Model file for the job. Use its own axes, mm. Give positions to 0.01 mm unless a question says otherwise; leave off trailing zeros. Write each loop counter-clockwise with the first axis right and the second up, starting at its lowest first coordinate (ties: lowest second). Pieces come first, ordered by that corner, then holes. Notation, with made-up numbers: (70.25, 46) - (75.25, 46) arc R28 ccw to (75.25, 79) - close; hole circle Ø10 at (72.5, 31.5). An arc over 180 degrees is marked (long way). Use CSV: the item, a comma, the result in double quotes.
Autodesk Inventor part; units mm, degrees
ref_plane "YZ Plane" through (0, 0, 0) normal (1, 0, 0) x (0, 1, 0)
ref_plane "XZ Plane" through (0, 0, 0) normal (0, 1, 0) x (-1, 0, 0)
ref_plane "XY Plane" through (0, 0, 0) normal (0, 0, 1) x (1, 0, 0)
sketch "Sketch1" plane through (0, 0, 0) normal (0, 0, 1) x (1, 0, 0)
  line L0 (0, 0) -> (380, 0)
  line L1 (380, 0) -> (380, 380)
  line L2 (380, 380) -> (0, 380)
  line L3 (0, 380) -> (0, 0)
  dimension "d0" = 380
  dimension "d1" = 380
extrude "Extrusion1" add sketch "Sketch1" along normal blind 380
sketch "Sketch2" plane through (0, 0, 380) normal (0, 0, 1) x (1, 0, 0)
  line L0 (30, 350) -> (350, 350)
  line L1 (350, 350) -> (350, 30)
  line L2 (350, 30) -> (30, 30)
  line L3 (30, 30) -> (30, 350)
  line L4 (380, 380) -> (0, 380)
  line L5 (0, 380) -> (0, 0)
  line L6 (0, 0) -> (380, 0)
  line L7 (380, 0) -> (380, 380)
  dimension "d4" = 30
  dimension "d5" = 30
  dimension "d6" = 30
  dimension "d7" = 30
extrude "Extrusion2" cut sketch "Sketch2" against normal blind 600 contours L0 L1 L2 L3
sketch "Sketch3" plane through (380, 0, 0) normal (1, 0, 0) x (0, 0, -1)
  line L0 (-350, 350) -> (-30, 350)
  line L1 (-30, 350) -> (-30, 30)
  line L2 (-30, 30) -> (-350, 30)
  line L3 (-350, 30) -> (-350, 350)
  line L4 (0, 380) -> (-380, 380)
  line L5 (-380, 0) -> (-380, 380)
  line L6 (0, 0) -> (0, 380)
  line L7 (0, 0) -> (-380, 0)
  dimension "d10" = 30
  dimension "d11" = 30
  dimension "d12" = 30
  dimension "d13" = 30
extrude "Extrusion3" cut sketch "Sketch3" against normal blind 600 contours L0 L1 L2 L3
sketch "Sketch4" plane through (0, 380, 0) normal (0, 1, 0) x (1, 0, 0)
  line L0 (30, -30) -> (30, 0)
  line L1 (350, -380) -> (350, -350)
  line L2 (30, -30) -> (350, -30)
  line L3 (350, -30) -> (350, -350)
  line L4 (350, -350) -> (30, -350)
  line L5 (30, -350) -> (30, -30)
  point P0 (0, 0)
extrude "Extrusion4" cut sketch "Sketch4" against normal blind 600
sketch "Sketch5" plane through (30, 0, 30) normal (1, 0, 0) x (0, 0, -1)
  line L0 (-350, 30) -> (-320, 30)
  line L1 (0, 30) -> (0, 0)
  line L2 (-320, 30) -> (0, 30)
  line L3 (0, 30) -> (0, 0)
  line L4 (0, 0) -> (-320, 0)
  line L5 (-320, 0) -> (-320, 30)
  point P0 (30, 0)
extrude "Extrusion5" add sketch "Sketch5" along normal blind 15
sketch "Sketch6" plane through (350, 0, 30) normal (0, 0, 1) x (1, 0, 0)
  line L0 (-320, 30) -> (-350, 30)
  line L1 (0, 30) -> (0, 0)
  line L2 (-320, 30) -> (0, 30)
  line L3 (0, 30) -> (0, 0)
  line L4 (0, 0) -> (-320, 0)
  line L5 (-320, 0) -> (-320, 30)
  point P0 (-350, 0)
extrude "Extrusion6" add sketch "Sketch6" along normal blind 15
sketch "Sketch7" plane through (350, 0, 350) normal (-1, 0, 0) x (0, 0, 1)
  line L0 (0, 30) -> (-320, 30)
  line L1 (0, 0) -> (-305, 0)
  line L2 (-320, 30) -> (0, 30)
  line L3 (0, 30) -> (0, 0)
  line L4 (0, 0) -> (-320, 0)
  line L5 (-320, 0) -> (-320, 30)
  point P0 (-350, 0)
extrude "Extrusion7" add sketch "Sketch7" along normal blind 15
sketch "Sketch8" plane through (45, 0, 350) normal (0, 0, -1) x (-1, 0, 0)
  line L0 (45, 0) -> (-335, 0)
  line L1 (-305, 30) -> (15, 30)
  line L2 (15, 30) -> (15, 0)
  line L3 (15, 0) -> (-305, 0)
  line L4 (-305, 0) -> (-305, 30)
  dimension "d24" = 320
extrude "Extrusion8" add sketch "Sketch8" along normal blind 15
sketch "Sketch9" plane through (0, 380, 0) normal (0, 1, 0) x (1, 0, 0)
  line L0 (0, -380) -> (380, -380)
  line L1 (0, 0) -> (20, 0)
  line L2 (10, -380) -> (0, -380)
  line L3 (0, -380) -> (0, 0)
  line L4 (20, 0) -> (380, 0)
  line L5 (380, 0) -> (380, -10)
  line L6 (380, -10) -> (10, -10)
  line L7 (10, -10) -> (10, -380)
  line L8 (0, -30) -> (0, -350)
  dimension "d27" = 10
  dimension "d28" = 10
extrude "Extrusion9" cut sketch "Sketch9" against normal blind 900
sketch "Sketch10" plane through (10, 380, 10) normal (0, 1, 0) x (1, 0, 0)
  line L0 (370, 0) -> (360, 0)
  line L1 (360, 0) -> (360, -370)
  line L2 (360, -370) -> (370, -370)
  line L3 (370, -370) -> (370, 0)
  line L4 (0, -370) -> (360, -370)
  line L5 (360, -370) -> (360, -360)
  line L6 (360, -360) -> (0, -360)
  line L7 (0, -360) -> (0, -370)
  point P0 (-10, 10)
  dimension "d31" = 10
  dimension "d32" = 10
extrude "Extrusion10" cut sketch "Sketch10" against normal blind 900
sketch "Sketch11" plane through (370, 380, 370) normal (1, 0, 0) x (0, 0, -1)
  line L0 (0, 0) -> (360, 0)
  line L1 (0, 0) -> (360, 0)
  line L2 (360, 0) -> (360, -10)
  line L3 (360, -10) -> (0, -10)
  line L4 (0, -10) -> (0, 0)
  line L5 (360, 0) -> (360, -380)
  line L6 (0, -380) -> (360, -380)
  line L7 (360, -380) -> (360, -370)
  line L8 (360, -370) -> (0, -370)
  line L9 (0, -370) -> (0, -380)
  point P0 (370, -380)
  dimension "d35" = 10
  dimension "d36" = 10
extrude "Extrusion11" cut sketch "Sketch11" against normal blind 900
sketch "Sketch13" plane through (10, 10, 370) normal (0, 0, 1) x (1, 0, 0)
  line L0 (0, 0) -> (360, 0)
  line L1 (360, 0) -> (260, 0)
  line L2 (260, 0) -> (260, 500)
  line L3 (260, 500) -> (360, 500)
  line L4 (360, 500) -> (360, 0)
  point P0 (-10, -10)
  point P1 (260, 0)
  dimension "d41" = 100
  dimension "d42" = 500
extrude "Extrusion13" add sketch "Sketch13" along normal blind 100
sketch "Sketch14" plane through (270, 510, 370) normal (0, 1, 0) x (1, 0, 0)
  line L0 (10, -10) -> (90, -10)
  line L1 (90, -10) -> (90, -90)
  line L2 (90, -90) -> (10, -90)
  line L3 (10, -90) -> (10, -10)
  line L4 (100, 0) -> (0, 0)
  line L5 (0, 0) -> (0, -100)
  line L6 (100, -100) -> (0, -100)
  line L7 (100, 0) -> (100, -100)
  point P0 (-270, 370)
  dimension "d45" = 10
  dimension "d46" = 10
  dimension "d47" = 10
  dimension "d48" = 10
extrude "Extrusion14" cut sketch "Sketch14" against normal blind 900 contours L0 L1 L2 L3
sketch "Sketch15" plane through (10, 10, 470) normal (0, 0, 1) x (1, 0, 0)
  line L0 (270, 500) -> (270, 0)
  line L1 (360, 20) -> (340, 20)
  line L2 (270, 490) -> (350, 490)
  line L3 (350, 490) -> (350, 20)
  line L4 (350, 20) -> (270, 20)
  line L5 (270, 20) -> (270, 490)
  line L6 (360, 500) -> (260, 500)
  point P0 (-10, -10)
  point P1 (270, 20)
  dimension "d51" = 10
extrude "Extrusion15" cut sketch "Sketch15" against normal blind 100
sketch "Sketch16" plane through (370, 10, 10) normal (1, 0, 0) x (0, 0, -1)
  line L0 (-450, 490) -> (-370, 490)
  line L1 (-370, 490) -> (-370, 20)
  line L2 (-370, 20) -> (-450, 20)
  line L3 (-450, 20) -> (-450, 490)
  line L4 (-360, 500) -> (-460, 500)
  line L5 (-460, 0) -> (-460, 500)
  line L6 (-360, 360) -> (-360, 500)
  line L7 (0, 0) -> (-460, 0)
  point P0 (10, -10)
  dimension "d54" = 10
  dimension "d55" = 10
  dimension "d56" = 10
  dimension "d57" = 20
extrude "Extrusion16" cut sketch "Sketch16" against normal blind 100
sketch "Sketch17" plane through (10, 10, 10) normal (0, -1, 0) x (1, 0, 0)
  line L0 (270, 450) -> (350, 450)
  line L1 (270, 370) -> (350, 370)
  line L2 (270, 450) -> (350, 450)
  line L3 (350, 450) -> (350, 370)
  line L4 (350, 370) -> (270, 370)
  line L5 (270, 370) -> (270, 450)
  point P0 (-10, -10)
  point P1 (350, 450)
extrude "Extrusion17" add sketch "Sketch17" against normal blind 20
sketch "Sketch19" plane through (370, 10, 10) normal (1, 0, 0) x (0, 0, -1)
  line L0 (-360, 500) -> (-460, 500)
  line L1 (-360, 490) -> (-360, 360)
  line L2 (-460, 500) -> (-360, 500)
  line L3 (-360, 500) -> (-360, 420)
  line L4 (-360, 420) -> (-460, 420)
  line L5 (-460, 420) -> (-460, 500)
  point P0 (10, -10)
  dimension "d65" = 80
extrude "Extrusion19" cut sketch "Sketch19" against normal blind 8900
sketch "Sketch20" plane through (370, 10, 10) normal (1, 0, 0) x (0, 0, -1)
  line L0 (-460, 420) -> (-450, 420)
  line L1 (-360, 360) -> (-360, 20)
  line L2 (-460, 420) -> (-360, 420)
  line L3 (-360, 420) -> (-360, 360)
  line L4 (-360, 360) -> (-460, 360)
  line L5 (-460, 360) -> (-460, 420)
  point P0 (10, -10)
extrude "Extrusion20" cut sketch "Sketch20" against normal blind 8900
sketch "Sketch21" plane through (270, 370, 380) normal (0, 0, 1) x (1, 0, 0)
  line L0 (10, -20) -> (10, 0)
  line L1 (0, 0) -> (10, 0)
  line L2 (10, 0) -> (10, -20)
  line L3 (10, -20) -> (0, -20)
  line L4 (0, -20) -> (0, 0)
  point P0 (-270, -370)
extrude "Extrusion21" add sketch "Sketch21" along normal up to surface (80 mm away)
sketch "Sketch22" plane through (280, 30, 470) normal (1, 0, 0) x (0, 0, -1)
  line L0 (0, 340) -> (10, 340)
  line L1 (10, 340) -> (10, 320)
  line L2 (10, 320) -> (0, 320)
  line L3 (0, 320) -> (0, 340)
  point P0 (470, -30)
  dimension "d72" = 20
extrude "Extrusion22" add sketch "Sketch22" along normal up to surface (80 mm away)
sketch "Sketch23" plane through (370, 10, 10) normal (1, 0, 0) x (0, 0, -1)
  line L0 (-370, 20) -> (-370, 360)
  line L1 (-450, 360) -> (-370, 360)
  line L2 (-370, 360) -> (-370, 340)
  line L3 (-370, 340) -> (-450, 340)
  line L4 (-450, 340) -> (-450, 360)
  point P0 (10, -10)
  dimension "d75" = 20
extrude "Extrusion23" add sketch "Sketch23" against normal blind 10
sketch "Sketch26" plane through (10, 10, 10) normal (0, -1, 0) x (1, 0, 0)
  line L0 (260, 460) -> (360, 460)
  line L1 (360, 0) -> (360, 460)
  line L2 (260, 460) -> (360, 460)
  line L3 (360, 460) -> (360, 360)
  line L4 (360, 360) -> (260, 360)
  line L5 (260, 360) -> (260, 460)
  point P0 (-10, -10)
  dimension "d86" = 100
extrude "Extrusion26" add sketch "Sketch26" along normal blind 120
sketch "Sketch30" plane through (10, 10, 470) normal (0, 0, 1) x (1, 0, 0)
  line L0 (360, 360) -> (260, 360)
  line L1 (260, 340) -> (260, 20)
  line L2 (360, 360) -> (260, 360)
  line L3 (260, 360) -> (260, 240)
  line L4 (260, 240) -> (360, 240)
  line L5 (360, 240) -> (360, 360)
  point P0 (-10, -10)
  dimension "d96" = 120
extrude "Extrusion30" cut sketch "Sketch30" against normal up to surface (100 mm away)
sketch "Sketch31" plane through (370, 10, 10) normal (1, 0, 0) x (0, 0, -1)
  line L0 (-450, 240) -> (-450, 20)
  line L1 (-450, 20) -> (-370, 20)
  line L2 (-370, 20) -> (-370, -110)
  line L3 (-370, -110) -> (-450, -110)
  line L4 (-450, -110) -> (-450, 20)
  line L5 (-360, -120) -> (-460, -120)
  point P0 (10, -10)
  dimension "d99" = 10
extrude "Extrusion31" cut sketch "Sketch31" against normal blind 200
sketch "Sketch32" plane through (10, 10, 470) normal (0, 0, 1) x (1, 0, 0)
  line L0 (350, 20) -> (270, 20)
  line L1 (270, 20) -> (350.1391, 20)
  line L2 (350.1391, 20) -> (350.1391, -110)
  line L3 (350.1391, -110) -> (270, -110)
  line L4 (270, -110) -> (270, 20)
  line L5 (360, -120) -> (260, -120)
  point P0 (-10, -10)
  point P1 (350, 20)
  dimension "d102" = 10
extrude "Extrusion32" cut sketch "Sketch32" against normal blind 100
sketch "Sketch33" plane through (270, 250, 380) normal (0, 0, 1) x (1, 0, 0)
  line L0 (0, 0) -> (10, 0)
  line L1 (10, -350) -> (10, 0)
  line L2 (0, 0) -> (10, 0)
  line L3 (10, 0) -> (10, -10)
  line L4 (10, -10) -> (0, -10)
  line L5 (0, -10) -> (0, 0)
  point P0 (-270, -250)
  dimension "d105" = 10
extrude "Extrusion33" add sketch "Sketch33" along normal up to surface (80 mm away)
sketch "Sketch34" plane through (280, 10, 370) normal (1, 0, 0) x (0, 0, -1)
  line L0 (-90, 240) -> (-90, 20)
  line L1 (-100, 240) -> (-90, 240)
  line L2 (-90, 240) -> (-90, 230)
  line L3 (-90, 230) -> (-100, 230)
  line L4 (-100, 230) -> (-100, 240)
  line L5 (0, 240) -> (-100, 240)
  line L6 (-10, 20) -> (-10, 240)
  line L7 (0, 240) -> (-10, 240)
  line L8 (-10, 240) -> (-10, 230)
  line L9 (-10, 230) -> (0, 230)
  line L10 (0, 230) -> (0, 240)
  point P0 (370, -10)
  point P1 (-90, 240)
  dimension "d108" = 10
extrude "Extrusion34" add sketch "Sketch34" along normal up to surface (90 mm away)
sketch "Sketch35" plane through (280, 250, 380) normal (0, 0, 1) x (1, 0, 0)
  line L0 (0, 0) -> (90, 0)
  line L1 (80, -10) -> (80, -220)
  line L2 (90, 0) -> (80, 0)
  line L3 (80, 0) -> (80, -10)
  line L4 (80, -10) -> (90, -10)
  line L5 (90, -10) -> (90, 0)
  point P0 (-280, -250)
extrude "Extrusion35" add sketch "Sketch35" along normal up to surface (80 mm away)
sketch "Sketch36" plane through (370, -100, 460) normal (0, 1, 0) x (1, 0, 0)
  line L0 (-340, 90) -> (-100, 90)
  line L1 (0, -10) -> (-100, -10)
  line L2 (-100, 90) -> (0, -10)
  circle A0 centre (-50, 40) radius 39
  point P0 (-370, 460)
  dimension "d113" = 78
extrude "Extrusion36" cut sketch "Sketch36" against normal blind 5
sketch "Sketch41" plane through (30, 350, 370) normal (0, 0, 1) x (1, 0, 0)
  point P0 (-30, -350)
sketch "Sketch42" plane through (270, 250, 470) normal (0, 1, 0) x (1, 0, 0)
  line L0 (-240, 100) -> (0, 100)
  line L1 (0, 100) -> (-10, 100)
  line L2 (-10, 100) -> (-10, 0)
  line L3 (-10, 0) -> (0, 0)
  line L4 (0, 0) -> (0, 100)
  point P0 (-270, 470)
  dimension "d119" = 10
extrude "Extrusion37" add sketch "Sketch42" against normal up to surface (360 mm away)
properties part number "Motor housing 2"
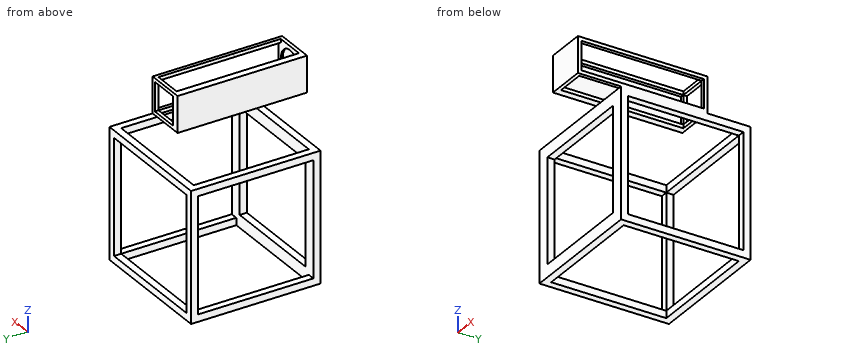
(1) Saw through at D-D, the plane z = 420. List the corners of the cut face in (x, y), then the cut area to 3 significant figures.
Checked values:
outline,"(260, -110) - (370, -110) - (370, -100) - (359, -100) - (359, -105) - (281, -105) - (281, -100) - (270, -100) - (270, 240) - (280, 240) - (280, 250) - (260, 250) - close; (360, 240) - (370, 240) - (370, 250) - (360, 250) - close"
area,"4,410 mm^2"
(2) Saw through at C-C, the plane x = 320. Count the separate pieces of the cut face and the enclosed holes in it, then the cut area to 3 significant figures.
Checked values:
separate pieces,"7"
enclosed holes,"0"
area,"3,010 mm^2"
(3) Saw through at A-A, the plane x = 212.5. List the corners of the cut face in (y, z).
Checked values:
outline,"(10, 10) - (30, 10) - (30, 45) - (10, 45) - close; (10, 335) - (30, 335) - (30, 370) - (10, 370) - close; (350, 10) - (370, 10) - (370, 30) - (350, 30) - close; (350, 350) - (370, 350) - (370, 370) - (350, 370) - close"
(4) Saw through at B-B, the plane z = 315. List the corners of the cut face in (x, y), then the cut area to 3 significant figures.
Checked values:
outline,"(10, 10) - (45, 10) - (45, 30) - (10, 30) - close; (10, 350) - (30, 350) - (30, 370) - (10, 370) - close; (335, 10) - (370, 10) - (370, 30) - (335, 30) - close; (350, 350) - (370, 350) - (370, 370) - (350, 370) - close"
area,"2,200 mm^2"
(5) Wall check: probe 1 along X at (y, z) = (-103.6, 420); probe 2 along Z at (x, y) = (320, -102); probe 3 along X at (y, z) = (3, 378). Give the ranges that are in metal, low to high. Write a range as [from, to].
Checked values:
probe 1,"x = [260, 281], [359, 370]"
probe 2,"z = [370, 381], [459, 470]"
probe 3,"x = [260, 280], [360.14, 370]"
(6) Flat gauge pins, fed straight in: P1, Ø2, axis at y = 179, z = 402, coming from the +X side; P2, Ø3, axis at y = 246, z = 426.5, coming from the -X side; P3, Ø12, axis at x = 259, y = 102, coming from the -Z side. Where does each tip first touch, or does it go through?
Checked values:
P1,"stops at x = 270"
P2,"stops at x = 260"
P3,"stops at z = 370"
